Check sheet for the modelled part. Datum: model origin and axes. Units: mm. A direction names the side the tool comes from. Give positions to 0.01 mm unless a question says otherwise; leave off trailing zeros. Order: outer loops, then holes, each group sorted by start corner. A loop starts at its lowest first (then second) coordinate and runs counter-clockwise, first axis right, second up.
```python
from build123d import *

# Parameters (mm, degrees)
SKIZZE1_W                       = 3.4
SKIZZE1_H                       = 1
AUFSATZ_LINEAR_AUSTRAGEN1_DEPTH = 3.81
SKIZZE3_W                       = 0.4
SKIZZE3_H                       = 0.4
AUFSATZ_LINEAR_AUSTRAGEN3_DEPTH = 0.5
SKIZZE4_W                       = 0.4
SKIZZE4_H                       = 0.4
AUFSATZ_LINEAR_AUSTRAGEN4_DEPTH = 1.915
SKIZZE5_W                       = 0.4
SKIZZE5_H                       = 0.4
AUFSATZ_LINEAR_AUSTRAGEN5_DEPTH = 1.915
SKIZZE6_W                       = 0.4
SKIZZE6_H                       = 0.4
AUFSATZ_LINEAR_AUSTRAGEN6_DEPTH = 3
FASE2_SIZE                      = 0.1
VERRUNDUNG1_R                   = 0.1
VERRUNDUNG2_R                   = 0.4


with BuildPart() as part:
    # Skizze1 → Aufsatz-Linear austragen1 (new body)
    with BuildSketch(Plane.XY):
        with Locations((1.7, 0.5)):
            Rectangle(SKIZZE1_W, SKIZZE1_H)
    extrude(amount=AUFSATZ_LINEAR_AUSTRAGEN1_DEPTH)

    # Skizze3 → Aufsatz-Linear austragen3 (add)
    with BuildSketch(Plane.XZ):
        with Locations((1.065, 3.175)):
            Rectangle(SKIZZE3_W, SKIZZE3_H)
        with Locations((2.335, 3.175)):
            Rectangle(SKIZZE3_W, SKIZZE3_H)
        with Locations((1.065, 1.905)):
            Rectangle(SKIZZE3_W, SKIZZE3_H)
        with Locations((2.335, 1.905)):
            Rectangle(SKIZZE3_W, SKIZZE3_H)
        with Locations((1.065, 0.635)):
            Rectangle(SKIZZE3_W, SKIZZE3_H)
        with Locations((2.335, 0.635)):
            Rectangle(SKIZZE3_W, SKIZZE3_H)
    extrude(amount=AUFSATZ_LINEAR_AUSTRAGEN3_DEPTH)

    # Skizze4 → Aufsatz-Linear austragen4 (add)
    with BuildSketch(Plane(origin=(2.535, 0, 0), x_dir=(0, 0, -1), z_dir=(1, 0, 0))):
        with Locations((-3.175, -0.3)):
            Rectangle(SKIZZE4_W, SKIZZE4_H)
        with Locations((-1.905, -0.3)):
            Rectangle(SKIZZE4_W, SKIZZE4_H)
        with Locations((-0.635, -0.3)):
            Rectangle(SKIZZE4_W, SKIZZE4_H)
    extrude(amount=AUFSATZ_LINEAR_AUSTRAGEN4_DEPTH)

    # Skizze5 → Aufsatz-Linear austragen5 (add)
    with BuildSketch(Plane.ZY.offset(-0.865)):
        with Locations((3.175, -0.3)):
            Rectangle(SKIZZE5_W, SKIZZE5_H)
        with Locations((1.905, -0.3)):
            Rectangle(SKIZZE5_W, SKIZZE5_H)
        with Locations((0.635, -0.3)):
            Rectangle(SKIZZE5_W, SKIZZE5_H)
    extrude(amount=AUFSATZ_LINEAR_AUSTRAGEN5_DEPTH)

    # Skizze6 → Aufsatz-Linear austragen6 (add)
    with BuildSketch(Plane(origin=(0, 1, 0), x_dir=(1, 0, 0), z_dir=(0, 1, 0))):
        with Locations((1.065, -0.635)):
            Rectangle(SKIZZE6_W, SKIZZE6_H)
        with Locations((2.335, -0.635)):
            Rectangle(SKIZZE6_W, SKIZZE6_H)
        with Locations((1.065, -1.905)):
            Rectangle(SKIZZE6_W, SKIZZE6_H)
        with Locations((2.335, -1.905)):
            Rectangle(SKIZZE6_W, SKIZZE6_H)
        with Locations((1.065, -3.175)):
            Rectangle(SKIZZE6_W, SKIZZE6_H)
        with Locations((2.335, -3.175)):
            Rectangle(SKIZZE6_W, SKIZZE6_H)
    extrude(amount=AUFSATZ_LINEAR_AUSTRAGEN6_DEPTH)

    # Fase2
    fase2_edges = [part.edges().sort_by_distance(p)[0] for p in [
        (4.45, -0.3, 0.835),
        (4.45, -0.5, 0.635),
        (4.45, -0.3, 0.435),
        (4.45, -0.1, 0.635),
        (-1.05, -0.3, 3.375),
        (-1.05, -0.1, 3.175),
        (-1.05, -0.3, 2.975),
        (-1.05, -0.5, 3.175),
        (-1.05, -0.3, 2.105),
        (-1.05, -0.1, 1.905),
        (-1.05, -0.3, 1.705),
        (-1.05, -0.5, 1.905),
        (-1.05, -0.3, 0.835),
        (-1.05, -0.1, 0.635),
        (-1.05, -0.3, 0.435),
        (-1.05, -0.5, 0.635),
        (1.265, 4, 0.635),
        (1.065, 4, 0.435),
        (0.865, 4, 0.635),
        (1.065, 4, 0.835),
        (2.535, 4, 0.635),
        (2.335, 4, 0.435),
        (2.135, 4, 0.635),
        (2.335, 4, 0.835),
        (1.265, 4, 1.905),
        (1.065, 4, 1.705),
        (0.865, 4, 1.905),
        (1.065, 4, 2.105),
        (2.535, 4, 1.905),
        (2.335, 4, 1.705),
        (2.135, 4, 1.905),
        (2.335, 4, 2.105),
        (1.265, 4, 3.175),
        (1.065, 4, 2.975),
        (0.865, 4, 3.175),
        (1.065, 4, 3.375),
        (2.535, 4, 3.175),
        (2.335, 4, 2.975),
        (2.135, 4, 3.175),
        (2.335, 4, 3.375),
        (4.45, -0.3, 3.375),
        (4.45, -0.5, 3.175),
        (4.45, -0.3, 2.975),
        (4.45, -0.1, 3.175),
        (4.45, -0.3, 2.105),
        (4.45, -0.5, 1.905),
        (4.45, -0.3, 1.705),
        (4.45, -0.1, 1.905),
    ]]
    chamfer(fase2_edges, length=FASE2_SIZE)

    # Verrundung1
    verrundung1_edges = [part.edges().sort_by_distance(p)[0] for p in [
        (0.865, -0.1, 3.175),
        (0.865, -0.1, 1.905),
        (0.865, -0.1, 0.635),
        (2.535, -0.1, 3.175),
        (2.535, -0.1, 1.905),
        (2.535, -0.1, 0.635),
    ]]
    fillet(verrundung1_edges, radius=VERRUNDUNG1_R - 0.0001)  # a hair under: the kernel refuses the full size

    # Verrundung2
    verrundung2_edges = [part.edges().sort_by_distance(p)[0] for p in [
        (1.265, -0.5, 3.175),
        (2.135, -0.5, 3.175),
        (1.265, -0.5, 1.905),
        (2.135, -0.5, 1.905),
        (1.265, -0.5, 0.635),
        (2.135, -0.5, 0.635),
    ]]
    fillet(verrundung2_edges, radius=VERRUNDUNG2_R)


solid = part.part
```
(1) Cross-section at A-A on x = 0.7. Enter the section's corners in (y, z) (3 decimals), then the cut area to 3 significant figures.
Response values:
outline: (-0.5, 0.435) - (-0.1, 0.435) - (-0.1, 0.835) - (-0.5, 0.835) - close; (-0.5, 1.705) - (-0.1, 1.705) - (-0.1, 2.105) - (-0.5, 2.105) - close; (-0.5, 2.975) - (-0.1, 2.975) - (-0.1, 3.375) - (-0.5, 3.375) - close; (0, 0) - (1, 0) - (1, 3.81) - (0, 3.81) - close
area: 4.29 mm2
(2) Material ranges on L1, parallel to Z at x = 2.3, y = 3.15 (3 decimals); L2, parallel to X at y = 3.35, z = 0.8 (3 decimals); L3, parallel to Y at x = 3.35, z = 0.25, recorded low to high.
Response values:
L1: z = 0.435 to 0.835, 1.705 to 2.105, 2.975 to 3.375
L2: x = 0.865 to 1.265, 2.135 to 2.535
L3: y = 0 to 1
(3) Cross-section at B-B on y = 2.1. Enter the section's corners in (x, z) (3 decimals).
Response values:
outline: (0.865, 0.435) - (1.265, 0.435) - (1.265, 0.835) - (0.865, 0.835) - close; (0.865, 1.705) - (1.265, 1.705) - (1.265, 2.105) - (0.865, 2.105) - close; (0.865, 2.975) - (1.265, 2.975) - (1.265, 3.375) - (0.865, 3.375) - close; (2.135, 0.435) - (2.535, 0.435) - (2.535, 0.835) - (2.135, 0.835) - close; (2.135, 1.705) - (2.535, 1.705) - (2.535, 2.105) - (2.135, 2.105) - close; (2.135, 2.975) - (2.535, 2.975) - (2.535, 3.375) - (2.135, 3.375) - close
(4) Gauge pin test, flat ends, axial feed: pin 1 Ø1.5 at (x, z) = (2, 2) entering from +Y; pin 2 Ø0.6 at (x, y) = (-0.5, -0.5) entering from -Z (3 decimals). Record the tip position at first contact, or that the pin passes through.
Response values:
pin 1: stops at y = 4
pin 2: stops at z = 0.435
(5) Cross-section at C-C on x = 3.9. Enter the section's corners in (y, z) (3 decimals), then the cut area to 3 significant figures.
Response values:
outline: (-0.5, 0.435) - (-0.1, 0.435) - (-0.1, 0.835) - (-0.5, 0.835) - close; (-0.5, 1.705) - (-0.1, 1.705) - (-0.1, 2.105) - (-0.5, 2.105) - close; (-0.5, 2.975) - (-0.1, 2.975) - (-0.1, 3.375) - (-0.5, 3.375) - close
area: 0.480 mm2
(6) Cross-section at D-D on z = 2.85. Enter the section's corners in (x, y), then the cut area to 3 significant figures.
Response values:
outline: (0, 0) - (3.4, 0) - (3.4, 1) - (0, 1) - close
area: 3.40 mm2
(7) Set-up check for faces 1 (the face through (3.4, 0.5, 1.9)), 2 (the face through (0, 0.5, 1.9)), 3 (the face through (1.7, 0, 1.9)): record each of +Z, -Z, +X, -X, +Y, -Y from which the full face is reachable in a straight line by a thin tool's end or side.
Response values:
face 1: +Z, -Z, +X, +Y
face 2: +Z, -Z, -X, +Y
face 3: none
